from build123d import *

# Parameters (mm, degrees)
SKETCH_1_R      = 10
SKETCH_1_W      = 41
SKETCH_1_H      = 4
EXTRUDE_1_DEPTH = 4
FILLET_3_R      = 3
FILLET_5_R      = 1


with BuildPart() as part:
    # Эскиз1 → Бобышка-Вытянуть1 (new body)
    with BuildSketch(Plane.XY):
        with BuildLine():
            Line((-26, -35), (26, -35))
            Line((26, -35), (26, -17))
            Line((26, -17), (14.402651465, 6.968761064))
            ThreePointArc((14.402651465, 6.968761064), (0, 16), (-14.402651465, 6.968761064))
            Line((-14.402651465, 6.968761064), (-26, -17))
            Line((-26, -17), (-26, -35))
        make_face()
        Circle(SKETCH_1_R, mode=Mode.SUBTRACT)
        with Locations((0, -27.5)):
            Rectangle(SKETCH_1_W, SKETCH_1_H, mode=Mode.SUBTRACT)
    extrude(amount=EXTRUDE_1_DEPTH)

    # Скругление3
    fillet_3_edges = [part.edges().sort_by_distance(p)[0] for p in [
        (-26, -35, 2),
        (-26, -17, 2),
        (26, -17, 2),
        (26, -35, 2),
    ]]
    fillet(fillet_3_edges, radius=FILLET_3_R)

    # Скругление5
    fillet_5_edges = [part.edges().sort_by_distance(p)[0] for p in [
        (-20.5, -25.5, 2),
        (-20.5, -29.5, 2),
        (20.5, -29.5, 2),
        (20.5, -25.5, 2),
    ]]
    fillet(fillet_5_edges, radius=FILLET_5_R)


solid = part.part
Read the model definition and answer for the solid it produces. Units are mm, in the model's axes. A direction names the side the tool comes from. Coordinates: 2 decimals unless noted, no trailing zeros. Order: outer loops, then holes, each group sorted by start corner. A loop starts at its lowest first (then second) coordinate and runs counter-clockwise, first axis right, second up. Notation, with made-up numbers: (46.5, 55.25) -> (71.5, 55.25) arc R15 cw to (71.5, 66.25) -> close; hole circle Ø1 at (62, 55). An arc over 180 degrees is marked (long way). Answer as a JSON object with one key per item and string values.
1) A tool of negligible diameter and unlimited length cuts with its end or side. For faces 1 (the face through (25.1, -34.14, 2.03)), 2 (the face through (0, -29.5, 2)), from which of +Z, -Z, +X, -X, +Y, -Y can it reach the whole face along a straight path? Write none if from no direction.
Model answer:
{"face 1": "+Z, -Z, +X, -Y", "face 2": "+Z, -Z"}
2) The mould has two halves that part along Y. Classify faces 3 (the face through (-20.5, -28, 2)), 4 (the face through (-2.17, -9.76, 1.97)), 5 (the face through (25.926, -17.027, 2.028)), 6 (the face through (26, -25, 2)): released by +Y, released by -Y, zero draft, split by the parting line, or undercut.
Model answer:
{"face 3": "undercut", "face 4": "undercut", "face 5": "released by +Y", "face 6": "zero draft"}
3) Consider line 1 along Y through (x, z) = (-0.5, 1.6); line 2 along X through (y, z) = (-26.5, 0.3); line 3 along Y through (x, z) = (-5, 0.8). Determine where each line is inside the solid, lowest interval first. Write a range as from..to.
Model answer:
{"line 1": "y = -35..-29.5, -25.5..-9.99, 9.99..15.99", "line 2": "x = -26..-20.5, 20.5..26", "line 3": "y = -35..-29.5, -25.5..-8.66, 8.66..15.2"}
4) A cutting plane is placed at B-B, the plane z = 1.9. Determine the outline of the cut face in (x, y), plus the area to 3 significant figures.
Model answer:
{"outline": "(-26, -32) arc R3 ccw to (-23, -35) -> (23, -35) arc R3 ccw to (26, -32) -> (26, -17.69) arc R3 ccw to (25.7, -16.38) -> (14.4, 6.97) arc R16 ccw to (-14.4, 6.97) -> (-25.7, -16.38) arc R3 ccw to (-26, -17.69) -> close; hole (-20.5, -28.5) arc R1 ccw to (-19.5, -29.5) -> (19.5, -29.5) arc R1 ccw to (20.5, -28.5) -> (20.5, -26.5) arc R1 ccw to (19.5, -25.5) -> (-19.5, -25.5) arc R1 ccw to (-20.5, -26.5) -> close; hole circle Ø20 at (0, 0)", "area": "1,610 mm²"}
5) A cutting plane is placed at A-A, the plane x = 0. Determine the outline of the cut face in (y, z), plus the area to 3 significant figures.
Model answer:
{"outline": "(-35, 0) -> (-29.5, 0) -> (-29.5, 4) -> (-35, 4) -> close; (-25.5, 0) -> (-10, 0) -> (-10, 4) -> (-25.5, 4) -> close; (10, 0) -> (16, 0) -> (16, 4) -> (10, 4) -> close", "area": "108 mm²"}
6) A cutting plane is placed at D-D, the plane x = -9. Determine the outline of the cut face in (y, z), plus the area to 3 significant figures.
Model answer:
{"outline": "(-35, 0) -> (-29.5, 0) -> (-29.5, 4) -> (-35, 4) -> close; (-25.5, 0) -> (-4.36, 0) -> (-4.36, 4) -> (-25.5, 4) -> close; (4.36, 0) -> (13.23, 0) -> (13.23, 4) -> (4.36, 4) -> close", "area": "142 mm²"}
7) Each of these flat-tipped pins is pushed along its axis until it touches: pin 1 (1.5 mm diameter, centred on x = -11.5, z = 1.5, fed in from +Y); pin 2 (2 mm diameter, centred on x = -2.5, z = 1, fed in from +Y). Where does it stop, or does it pass through?
Model answer:
{"pin 1": "stops at y = 11.85", "pin 2": "stops at y = 15.93"}
8) A cutting plane is placed at C-C, the plane y = 0. Determine the outline of the cut face in (x, z), plus the area to 3 significant figures.
Model answer:
{"outline": "(-17.77, 0) -> (-10, 0) -> (-10, 4) -> (-17.77, 4) -> close; (10, 0) -> (17.77, 0) -> (17.77, 4) -> (10, 4) -> close", "area": "62.2 mm²"}
